Verification items for the finished model (mm, model axes). Face numbers are marked on the shaded views. A direction names the side the tool comes from. Round coordinates to 2 decimals unless told otherwise and drop trailing zeros. Write each loop counter-clockwise with the first axis right and the second up, starting at its lowest first coordinate (ties: lowest second). Pieces come first, ordered by that corner, then holes. Notation, with made-up numbers: (-28, 78.5) - (21, 78.5) arc R5 ccw to (21, 86.5) - close; hole circle Ø11 at (-22, 77.5). An arc over 180 degrees is marked (long way). Answer as a JSON object with one key per item and string values. Group by question number.
1) Go/stop test with flat-tipped pins: pin 1 Ø4 at (x, y) = (5.5, -5.5) entering from +Z; pin 2 Ø1.5 at (x, z) = (4.5, 1) entering from -Y. Record where each tip stops, or that it passes through.
2) Section check B-B (z = 1). Enter the section's corners in (x, y) (3 decimals).
3) Mould release check, pull along Y, two halves, no side actions. Record for the marked faces 1, 2 and 3: +Y half, -Y half, draft (parallel to the pull), parting line (faces both ways), or undercut.
4) Section check D-D (y = -6.75). Enter the section's corners in (x, z).
5) Section check C-C (x = 4.75). Enter the section's corners in (y, z).
6) Thickness scan on line 1 (Y direction, x = -2, z = 1) (3 decimals); line 2 (Y direction, x = 4.75, z = 2); line 3 (X direction, y = 5.75, z = 2.5). Record the ranges inside material, lowest first.
7) Set-up check for the marked faces 4, 5 and 6: record each of +Z, -Z, +X, -X, +Y, -Y from which the full face is reachable in a straight line by a thin tool's end or side.
8) Section check A-A (y = 3.25). Enter the section's corners in (x, z) (3 decimals).
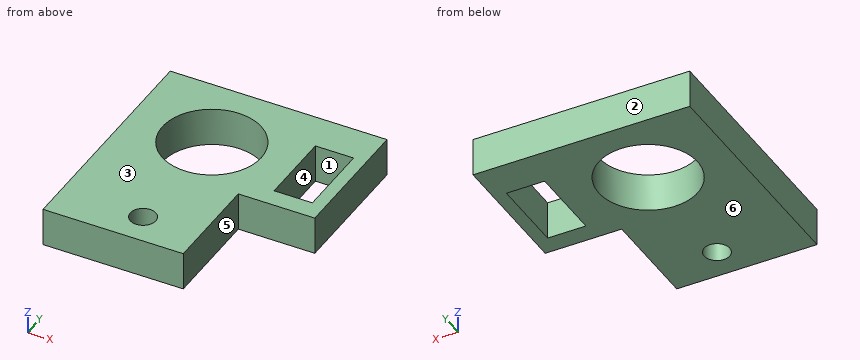
```python
from build123d import *

# Parameters (mm, degrees)
BOSS_EXTRUDE3_DEPTH = 3
SKETCH6_W           = 3
SKETCH6_H           = 6
CUT_EXTRUDE2_DEPTH  = 3
SKETCH7_R           = 3.875
SKETCH7_R_2         = 1
CUT_EXTRUDE3_DEPTH  = 3


with BuildPart() as part:
    # Sketch3 → Boss-Extrude3 (new body)
    with BuildSketch(Plane.XY):
        Polygon((2.5, -9.25), (2.5, -1.25), (8.5, -1.25), (8.5, 9.25), (-8.5, 9.25), (-8.5, -9.25), align=None)
    extrude(amount=BOSS_EXTRUDE3_DEPTH)

    # Sketch6 → Cut-Extrude2 (cut)
    with BuildSketch(Plane.XY.offset(3)):
        with Locations((6, 3.25)):
            Rectangle(SKETCH6_W, SKETCH6_H)
    extrude(amount=-CUT_EXTRUDE2_DEPTH, mode=Mode.SUBTRACT)

    # Sketch7 → Cut-Extrude3 (cut)
    with BuildSketch(Plane.XY.offset(3)):
        with Locations((-2, 3.25)):
            Circle(SKETCH7_R)
        with Locations((-2, -6.75)):
            Circle(SKETCH7_R_2)
    extrude(amount=-CUT_EXTRUDE3_DEPTH, mode=Mode.SUBTRACT)


solid = part.part
```
Returned:
{
 "1": {"pin 1": "through", "pin 2": "y = -1.25"},
 "2": {"outline": "(-8.5, -9.25) - (2.5, -9.25) - (2.5, -1.25) - (8.5, -1.25) - (8.5, 9.25) - (-8.5, 9.25) - close; hole circle Ø7.75 at (-2, 3.25); hole circle Ø2 at (-2, -6.75); hole (4.5, 0.25) - (7.5, 0.25) - (7.5, 6.25) - (4.5, 6.25) - close"},
 "3": {"face 1": "undercut", "face 2": "+Y half", "face 3": "draft"},
 "4": {"outline": "(-8.5, 0) - (-3, 0) - (-3, 3) - (-8.5, 3) - close; (-1, 0) - (2.5, 0) - (2.5, 3) - (-1, 3) - close"},
 "5": {"outline": "(-1.25, 0) - (0.25, 0) - (0.25, 3) - (-1.25, 3) - close; (6.25, 0) - (9.25, 0) - (9.25, 3) - (6.25, 3) - close"},
 "6": {"line 1": "-9.25 to -7.75, -5.75 to -0.625, 7.125 to 9.25", "line 2": "-1.25 to 0.25, 6.25 to 9.25", "line 3": "-8.5 to -4.96, 0.96 to 4.5, 7.5 to 8.5"},
 "7": {"face 4": "+Z, -Z", "face 5": "+Z, -Z, +X, -Y", "face 6": "-Z, +X, -X, +Y, -Y"},
 "8": {"outline": "(-8.5, 0) - (-5.875, 0) - (-5.875, 3) - (-8.5, 3) - close; (1.875, 0) - (4.5, 0) - (4.5, 3) - (1.875, 3) - close; (7.5, 0) - (8.5, 0) - (8.5, 3) - (7.5, 3) - close"}
}
